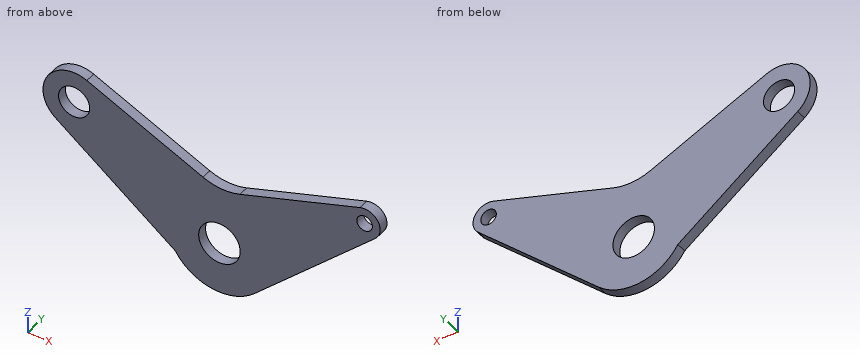
```python
from build123d import *

# Parameters (mm, degrees)
F0_R     = 2
F0_R_2   = 1.5
F0_R_3   = 0.75
F1_DEPTH = 0.5


with BuildPart() as f1:
    # F0 (on Front) → F1 (new body, symmetric)
    with BuildSketch(Plane.XZ):
        with BuildLine():
            Line((-24.761863, 14.850086), (-35.955657, 19.889062))
            ThreePointArc((-35.955657, 19.889062), (-39.773049, 18.674288), (-38.979378, 14.74768))
            Line((-38.979378, 14.74768), (-27.427554, 6.141753))
            ThreePointArc((-27.427554, 6.141753), (-23.858251, 3.820055), (-19.794239, 5.090492))
            Line((-19.794239, 5.090492), (-8.168313, 15.766349))
            ThreePointArc((-8.168313, 15.766349), (-7.88459, 17.622506), (-9.635309, 18.301331))
            Line((-9.635309, 18.301331), (-21.201303, 14.642294))
            ThreePointArc((-21.201303, 14.642294), (-23.000741, 14.417917), (-24.761863, 14.850086))
        make_face()
        with Locations((-23.17609, 8.773302)):
            Circle(F0_R, mode=Mode.SUBTRACT)
        with Locations((-37.18711, 17.153459)):
            Circle(F0_R_2, mode=Mode.SUBTRACT)
        with Locations((-9.182868, 16.871192)):
            Circle(F0_R_3, mode=Mode.SUBTRACT)
    extrude(amount=F1_DEPTH, both=True)


solid = f1.part
```
Read the model definition and answer for the solid it produces. Units are mm, in the model's axes. Give positions to 0.01 mm unless a question says otherwise; leave off trailing zeros. Order: outer loops, then holes, each group sorted by start corner. A loop starts at its lowest first (then second) coordinate and runs counter-clockwise, first axis right, second up.
(1) Find section D-D (x = -18). Give the vertices of the cut face in (y, z), plus the area to 3 significant figures.
(2) Find section A-A (z = 9.25). Give the vertices of the cut face in (x, y).
(3) Find section B-B (x = -37). Give the vertices of the cut face in (y, z), plus the area to 3 significant figures.
(4) Find section C-C (y = -0.35). Give the vertices of the cut face in (x, z).
(5) Given pin 1 (2 mm diameter, centred on x = -9.18, z = 16.87, fed in from +Y), flat-ended and moving along its own axis, determine where the tip first touches the part or whether it passes through.
(6) Straight lines are drawn through the part: L1, parallel to X at y = -0.4, z = 10; L2, parallel to Z at x = -25, y = -0.4; L3, parallel to X at y = -0.1, z = 18.5. For each, find the intervals that lie inside material, in ascending order.
Result sheet:
1. outline: (-0.5, 6.74) - (0.5, 6.74) - (0.5, 15.66) - (-0.5, 15.66) - close
1. area: 8.92 mm2
2. outline: (-31.6, -0.5) - (-25.12, -0.5) - (-25.12, 0.5) - (-31.6, 0.5) - close; (-21.23, -0.5) - (-15.26, -0.5) - (-15.26, 0.5) - (-21.23, 0.5) - close
3. outline: (-0.5, 13.27) - (0.5, 13.27) - (0.5, 15.67) - (-0.5, 15.67) - close; (-0.5, 18.64) - (0.5, 18.64) - (0.5, 20.15) - (-0.5, 20.15) - close
3. area: 3.90 mm2
4. outline: (-38.98, 14.75) - (-27.43, 6.14) arc R5 ccw to (-19.79, 5.09) - (-8.17, 15.77) arc R1.5 ccw to (-9.64, 18.3) - (-21.2, 14.64) arc R5 cw to (-24.76, 14.85) - (-35.96, 19.89) arc R3 ccw to start; hole circle Ø3 at (-37.19, 17.15); hole circle Ø4 at (-23.18, 8.77); hole circle Ø1.5 at (-9.18, 16.87)
5. pin 1: stops at y = 0.5
6. L1: x = -32.61 to -24.76, -21.6 to -14.45
6. L2: z = 4.12 to 7.95, 9.59 to 14.96
6. L3: x = -39.87 to -37.85, -36.53 to -32.87
